Can you work these out from the drawing? Everything is in mm from the part's minimum corner. A direction names the side the tool comes from. Coordinates: 2 decimals unless noted, no trailing zeros. Loops run counter-clockwise (first coordinate to the right, second up) from the corner with the lowest first, then second, coordinate; pieces in that order, holes last.
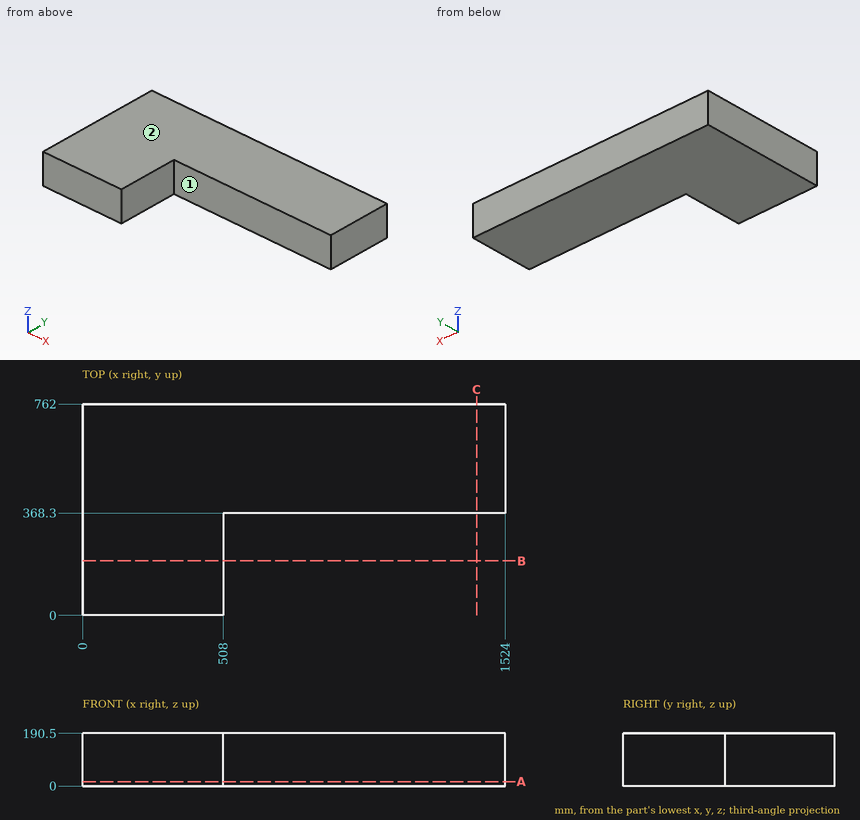
1. On a 3-axis mill with a long thin cutter (end or side, diameter ignored), from which of +Z, -Z, +X, -X, +Y, -Y can I reach the whole of each face in a straight line? I mean the marked faces 1 and 2. Say none if no direction works.
2. I want a section at C-C (x = 1421.5). Please give me the cut outline in (y, z), then the cut area to 3 significant figures.
3. I need wall thicknesses on line 1 along X through (y, z) = (254.5, 148); line 2 along Y through (x, z) = (976, 30.5). Which ranges of each line are inside material? Lowest first, please.
4. I want a section at B-B (y = 196.5). Please give me the cut outline in (x, z).
5. I want a section at A-A (z = 16). Please give me the cut outline in (x, y).
Response values:
1. face 1: +Z, -Z, +X, -Y
1. face 2: +Z, +X, -X, +Y, -Y
2. outline: (368.3, 0) - (762, 0) - (762, 190.5) - (368.3, 190.5) - close
2. area: 75,000 mm2
3. line 1: x = 0 to 508
3. line 2: y = 368.3 to 762
4. outline: (0, 0) - (508, 0) - (508, 190.5) - (0, 190.5) - close
5. outline: (0, 0) - (508, 0) - (508, 368.3) - (1524, 368.3) - (1524, 762) - (0, 762) - close
